from build123d import *

# Parameters (mm, degrees)
F0_W     = 63.5
F0_H     = 38.1
F1_DEPTH = 6.35
F2_W     = 50.8
F2_H     = 6.35
F3_DEPTH = 31.75
F5_DEPTH = 6.35
F7_DEPTH = 12.7


with BuildPart() as f1:
    # F0 (on Top) → F1 (new body)
    with BuildSketch(Plane.XY):
        Rectangle(F0_W, F0_H)
    extrude(amount=F1_DEPTH)

    # F2 (on face) → F3 (join)
    with BuildSketch(Plane.XY.offset(6.35)):
        with Locations((-6.35, 15.875)):
            Rectangle(F2_W, F2_H)
    extrude(amount=F3_DEPTH)

    # F4 (on face) → F5 (join)
    with BuildSketch(Plane.YZ.offset(31.75)):
        Polygon((-19.05, 6.35), (12.7, 6.35), (-19.05, 38.1), align=None)
    extrude(amount=-F5_DEPTH)

    # F6 (on face) → F7 (cut)
    with BuildSketch(Plane.YZ.offset(31.75)):
        Polygon((19.05, 6.35), (12.7, 6.35), (19.05, 0), align=None)
    extrude(amount=-F7_DEPTH, mode=Mode.SUBTRACT)


solid = f1.part
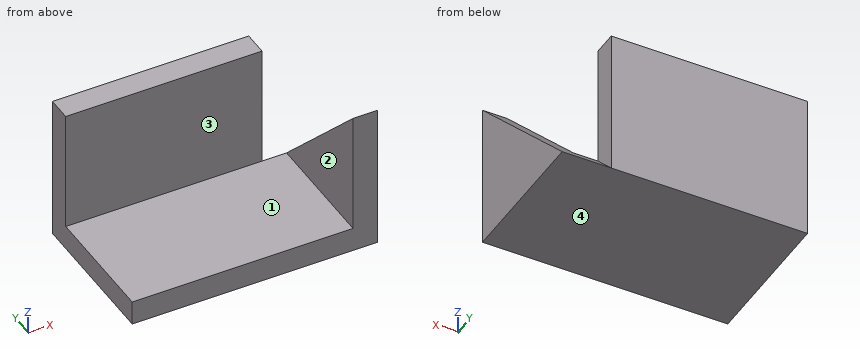
Geometry: final body of the model. Coordinates: model frame, mm. Face numbers are marked on the shaded views. A direction names the side the tool comes from. Give positions to 0.01 mm unless a question says otherwise; leave off trailing zeros. Write each loop counter-clockwise with the first axis right and the second up, starting at its lowest first coordinate (ties: lowest second). Pieces come first, ordered by that corner, then holes.
(1) Access query for the marked faces 1, 2, 3 and 4. Directions: +Z, -Z, +X, -X, +Y, -Y. A direction counts if a zero-diameter tool reaches every point of the face in a straight line with its end or side. Return the directions, or none.
(2) Cut plane B-B, the plane y = 14. Return loops of the section in (x, z), then the cut area to 3 significant figures.
(3) First-contact query: P1, Ø9.5, axis at x = 0, z = 21, coming from the -Y side; P2, Ø16, axis at y = -10, z = 26, coming from the -X side; P3, Ø6, axis at x = 7.5, y = -11, coming from the +Z side. Flat tips, straight axial feed; report the tip coordinate or a pass-through.
(4) Cut plane D-D, the plane x = -21. Return loops of the section in (y, z).
(5) Cut plane A-A, the plane z = 8. Return loops of the section in (x, y).
(6) Ray query, line 1 (Z direction, x = -22, y = -6); line 2 (X direction, y = -11, z = 11); line 3 (Y direction, x = -17, z = 25.5). Return the intervals inside material, ascending.
(7) Cut plane C-C, the plane z = 23. Return loops of the section in (x, y).
Values follow:
1. face 1: +Z, -X, -Y
1. face 2: +Z, -X, +Y, -Y
1. face 3: +Z, +X, -X, -Y
1. face 4: -Z, +X, -X, +Y, -Y
2. outline: (-31.75, 0) - (31.75, 0) - (31.75, 5.05) - (19.05, 5.05) - (19.05, 38.1) - (-31.75, 38.1) - close
2. area: 2,000 mm2
3. P1: stops at y = 12.7
3. P2: stops at x = 25.4
3. P3: stops at z = 6.35
4. outline: (-19.05, 0) - (19.05, 0) - (19.05, 38.1) - (12.7, 38.1) - (12.7, 6.35) - (-19.05, 6.35) - close
5. outline: (-31.75, 12.7) - (19.05, 12.7) - (19.05, 19.05) - (-31.75, 19.05) - close; (25.4, -19.05) - (31.75, -19.05) - (31.75, 11.05) - (25.4, 11.05) - close
6. line 1: z = 0 to 6.35
6. line 2: x = 25.4 to 31.75
6. line 3: y = 12.7 to 19.05
7. outline: (-31.75, 12.7) - (19.05, 12.7) - (19.05, 19.05) - (-31.75, 19.05) - close; (25.4, -19.05) - (31.75, -19.05) - (31.75, -3.95) - (25.4, -3.95) - close
